```python
from build123d import *

# Parameters (mm, degrees)
F1_DEPTH = 3.175
F2_DEPTH = 25.4
F3_DEPTH = 25.4


with BuildPart() as f1:
    # F0 (on Top) → F1 (new body)
    with BuildSketch(Plane.XY):
        with BuildLine():
            ThreePointArc((98.425, 149.3462514694), (50.8, 130.1850769842), (3.175, 149.3462514694))
            Line((3.175, 149.3462514694), (3.175, 3.3780224621))
            Line((3.175, 3.3780224621), (3.175, 0.2030224621))
            Line((3.175, 0.2030224621), (98.425, 0.2030224621))
            Line((98.425, 0.2030224621), (98.425, 3.3780224621))
            Line((98.425, 3.3780224621), (98.425, 149.3462514694))
        make_face()
    extrude(amount=F1_DEPTH)

    # F0 (on Top) → F2 (join)
    with BuildSketch(Plane.XY):
        with BuildLine():
            ThreePointArc((3.175, 149.3462514694), (1.5605666607, 150.9483798686), (0, 152.6030224621))
            Line((0, 152.6030224621), (0, 0.2030224621))
            Line((0, 0.2030224621), (3.175, 0.2030224621))
            Line((3.175, 0.2030224621), (3.175, 3.3780224621))
            Line((3.175, 3.3780224621), (3.175, 149.3462514694))
        make_face()
    extrude(amount=F2_DEPTH)

    # F0 (on Top) → F3 (join)
    with BuildSketch(Plane.XY):
        with BuildLine():
            ThreePointArc((101.6, 152.6030224621), (100.0394333393, 150.9483798686), (98.425, 149.3462514694))
            Line((98.425, 149.3462514694), (98.425, 3.3780224621))
            Line((98.425, 3.3780224621), (98.425, 0.2030224621))
            Line((98.425, 0.2030224621), (101.6, 0.2030224621))
            Line((101.6, 0.2030224621), (101.6, 152.6030224621))
        make_face()
    extrude(amount=F3_DEPTH)


solid = f1.part
```
Here's how the part is built. I have some questions about the finished solid (model axes, mm). A direction names the side the tool comes from. Give positions to 0.01 mm unless a question says otherwise; leave off trailing zeros. Order: outer loops, then holes, each group sorted by start corner. A loop starts at its lowest first (then second) coordinate and runs counter-clockwise, first axis right, second up. Notation, with made-up numbers: (89.5, 62) - (93.5, 62) arc R18 ccw to (93.5, 83) - close; hole circle Ø8 at (-30, -25). An arc over 180 degrees is marked (long way). Answer as a JSON object with one key per item and string values. Group by question number.
Item 1: Which directions (+Z, -Z, +X, -X, +Y, -Y) give clear straight access to the entire face, cutting with the end or side of a thin tool? Please do faces 1 (the flat face through (50, 76, 3.175)), 2 (the flat face through (50, 77, 0)).
Item 2: If we section it at D-D on x = 74: Please give me the cut outline in (y, z) (3 decimals).
Item 3: If we section it at C-C on x = 52: Please give me the cut outline in (y, z) (3 decimals), and give its area (3 significant figures).
Item 4: If we section it at B-B on y = 120: Please give me the cut outline in (x, z) (3 decimals), and give its area (3 significant figures).
Item 5: If we mould it in two halves opening along X, with no side actions, what happens to faces 3 (the flat face through (0, 77, 13)), 4 (the flat face through (101.6, 75, 13)), 5 (the flat face through (98.425, 76, 14))? For each: pulls with the +X half, pulls with the -X half, needs draft (parallel to the pull), parting line crosses it, or undercut.
Item 6: If we section it at A-A on z = 8: Please give me the cut outline in (x, y) (1 decimal), and give its area (3 significant figures).
Item 7: Please list where these lines run through material, in increasing order: probe 1 along X at (y, z) = (130, 6) (3 decimals); probe 2 along Z at (x, y) = (40, 105) (3 decimals).
Result set:
{
 "1": {"face 1": "+Z, +Y, -Y", "face 2": "-Z, +X, -X, +Y, -Y"},
 "2": {"outline": "(0.203, 0) - (134.217, 0) - (134.217, 3.175) - (0.203, 3.175) - close"},
 "3": {"outline": "(0.203, 0) - (130.196, 0) - (130.196, 3.175) - (0.203, 3.175) - close", "area": "413 mm²"},
 "4": {"outline": "(0, 0) - (101.6, 0) - (101.6, 25.4) - (98.425, 25.4) - (98.425, 3.175) - (3.175, 3.175) - (3.175, 25.4) - (0, 25.4) - close", "area": "464 mm²"},
 "5": {"face 3": "pulls with the -X half", "face 4": "pulls with the +X half", "face 5": "undercut"},
 "6": {"outline": "(0, 0.2) - (3.2, 0.2) - (3.2, 149.3) arc R68.8 cw to (0, 152.6) - close; (98.4, 0.2) - (101.6, 0.2) - (101.6, 152.6) arc R68.8 cw to (98.4, 149.3) - close", "area": "957 mm²"},
 "7": {"probe 1": "0 to 3.175, 98.425 to 101.6", "probe 2": "0 to 3.175"}
}
